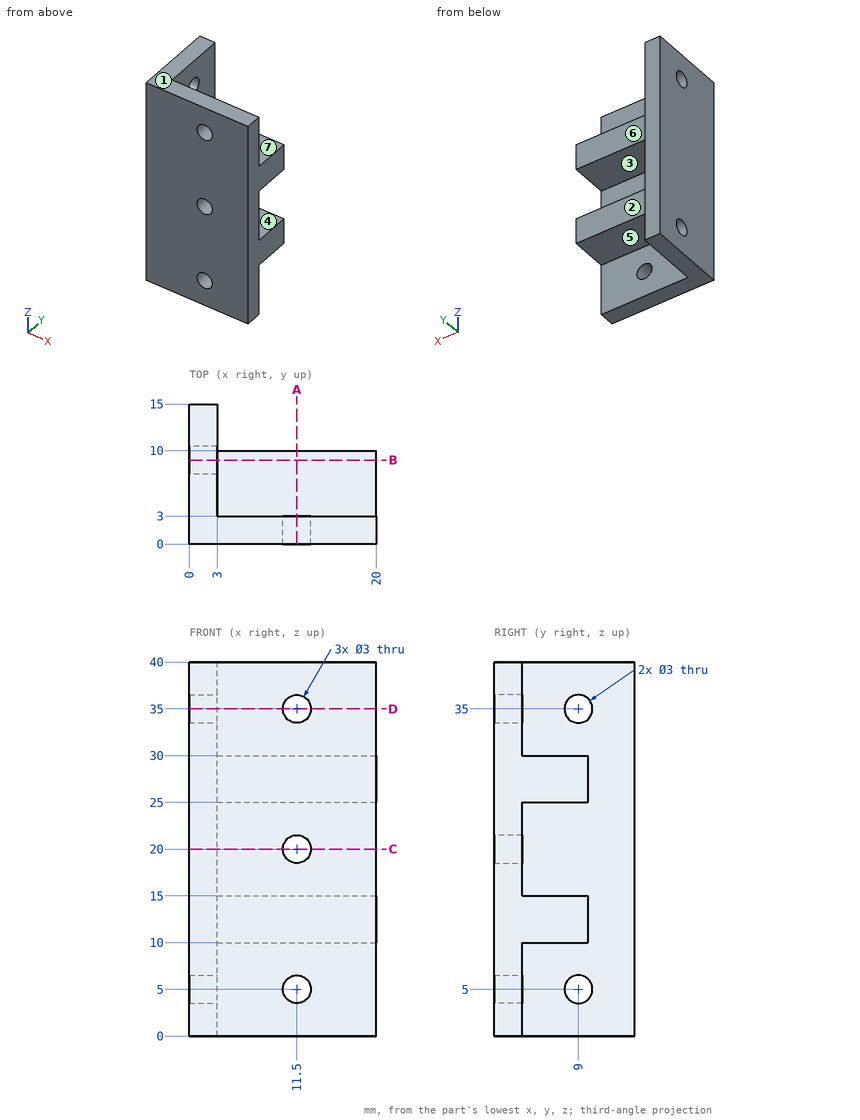
Source: three-view drawing plus pictorial views. Frame: mm from the lowest corner of the part. A direction names the side the tool comes from. Give positions to 0.01 mm unless a question says otherwise; leave off trailing zeros. Order: outer loops, then holes, each group sorted by start corner. A loop starts at its lowest first (then second) coordinate and runs counter-clockwise, first axis right, second up. Notation, with made-up numbers: M 67,34.25 L 112,34.25 A27 ccw 112,71.25 Z; hole C -5.75,56 d11. An arc over 180 degrees is marked long. Return JSON: item names as keys, results as strings.
1) Section query C-C on z = 20. Output: boundary loops of the cut face in (x, y), and give its area (3 significant figures).
Taken from the geometry:
{"outline": "M 0,0 L 10,0 L 10,3 L 3,3 L 3,15 L 0,15 Z; M 13,0 L 20,0 L 20,3 L 13,3 Z", "area": "87.0 mm2"}
2) Mould query, pull axis Z, two halves, no side actions, for the marked faces 1, 2 and 3. Classes: released by +Z, released by -Z, zero draft, split by the parting line, or undercut.
Taken from the geometry:
{"face 1": "released by +Z", "face 2": "zero draft", "face 3": "undercut"}
3) Section query B-B on y = 9. Output: boundary loops of the cut face in (x, z).
Taken from the geometry:
{"outline": "M 0,0 L 3,0 L 3,3.5 L 0,3.5 Z; M 0,6.5 L 3,6.5 L 3,10 L 20,10 L 20,15 L 3,15 L 3,25 L 20,25 L 20,30 L 3,30 L 3,33.5 L 0,33.5 Z; M 0,36.5 L 3,36.5 L 3,40 L 0,40 Z"}
4) Section query D-D on z = 35. Output: boundary loops of the cut face in (x, y).
Taken from the geometry:
{"outline": "M 0,0 L 10,0 L 10,3 L 3,3 L 3,7.5 L 0,7.5 Z; M 0,10.5 L 3,10.5 L 3,15 L 0,15 Z; M 13,0 L 20,0 L 20,3 L 13,3 Z"}
5) Section query A-A on x = 11.5. Output: boundary loops of the cut face in (y, z).
Taken from the geometry:
{"outline": "M 0,0 L 3,0 L 3,3.5 L 0,3.5 Z; M 0,6.5 L 3,6.5 L 3,10 L 10,10 L 10,15 L 3,15 L 3,18.5 L 0,18.5 Z; M 0,21.5 L 3,21.5 L 3,25 L 10,25 L 10,30 L 3,30 L 3,33.5 L 0,33.5 Z; M 0,36.5 L 3,36.5 L 3,40 L 0,40 Z"}
6) Contact query for flat-ended pins moving along their axis: pin 1 (3 mm diameter, centred on x = 4, y = 3.5, fed in from -Z); pin 2 (5.5 mm diameter, centred on x = 12, y = 7.5, fed in from -Z); pin 3 (2 mm diameter, centred on y = 13, z = 9, fed in from +X); pin 4 (2.5 mm diameter, centred on x = 12.5, z = 12.5, fed in from +Y). Output: stop coordinate, or through.
Taken from the geometry:
{"pin 1": "stops at z = 0", "pin 2": "stops at z = 10", "pin 3": "stops at x = 3", "pin 4": "stops at y = 10"}
7) Access query for the marked faces 4, 5, 6 and 7. Directions: +Z, -Z, +X, -X, +Y, -Y. A direction counts if a zero-diameter tool reaches every point of the face in a straight line with its end or side. Return the directions, or none.
Taken from the geometry:
{"face 4": "+X, +Y", "face 5": "-Z, +X, +Y", "face 6": "+Z, -Z, +X, +Y", "face 7": "+Z, +X, +Y"}
8) Line query: L1, parallel to Z at x = 1.65, y = 9; L2, parallel to X at y = 2, z = 5; L3, parallel to Z at x = 16.25, y = 7.25. Output: solid intervals per line, ascending. Write a range as [from, to].
Taken from the geometry:
{"L1": "z = [0, 3.5], [6.5, 33.5], [36.5, 40]", "L2": "x = [0, 10], [13, 20]", "L3": "z = [10, 15], [25, 30]"}
